Check sheet for the drawn part. Datum: minimum x, y, z corner. Units: mm. A direction names the side the tool comes from. Round coordinates to 2 decimals unless told otherwise and drop trailing zeros. Write each loop counter-clockwise with the first axis right and the second up, starting at its lowest first coordinate (ties: lowest second). Pieces come first, ordered by that corner, then holes.
Item 1: Tool access check on the marked faces 1, 2 and 3. Record the directions out of +Z, -Z, +X, -X, +Y, -Y that give a thin tool (end or side, any length) a straight path to the whole face; none if there is none.
Item 2: Cross-section at C-C on x = 38. Enter the section's corners in (y, z).
Item 3: Cross-section at D-D on x = 26. Enter the section's corners in (y, z), plus the area to 3 significant figures.
Item 4: Material ranges on line 1 (Z direction, x = 45, y = 4.75); line 2 (X direction, y = 4.5, z = 25.75), recorded low to high.
Item 5: Go/stop test with flat-tipped pins: pin 1 Ø10 at (y, z) = (10.5, 17.5) entering from +X; pin 2 Ø2 at (y, z) = (10.5, 13.5) entering from -X; pin 3 Ø0.5 at (y, z) = (15, 27.5) entering from -X. Record where each tip stops, or that it passes through.
Item 6: Cross-section at A-A on y = 18.5. Enter the section's corners in (x, z).
Item 7: Cross-section at B-B on z = 14.5. Enter the section's corners in (x, y).
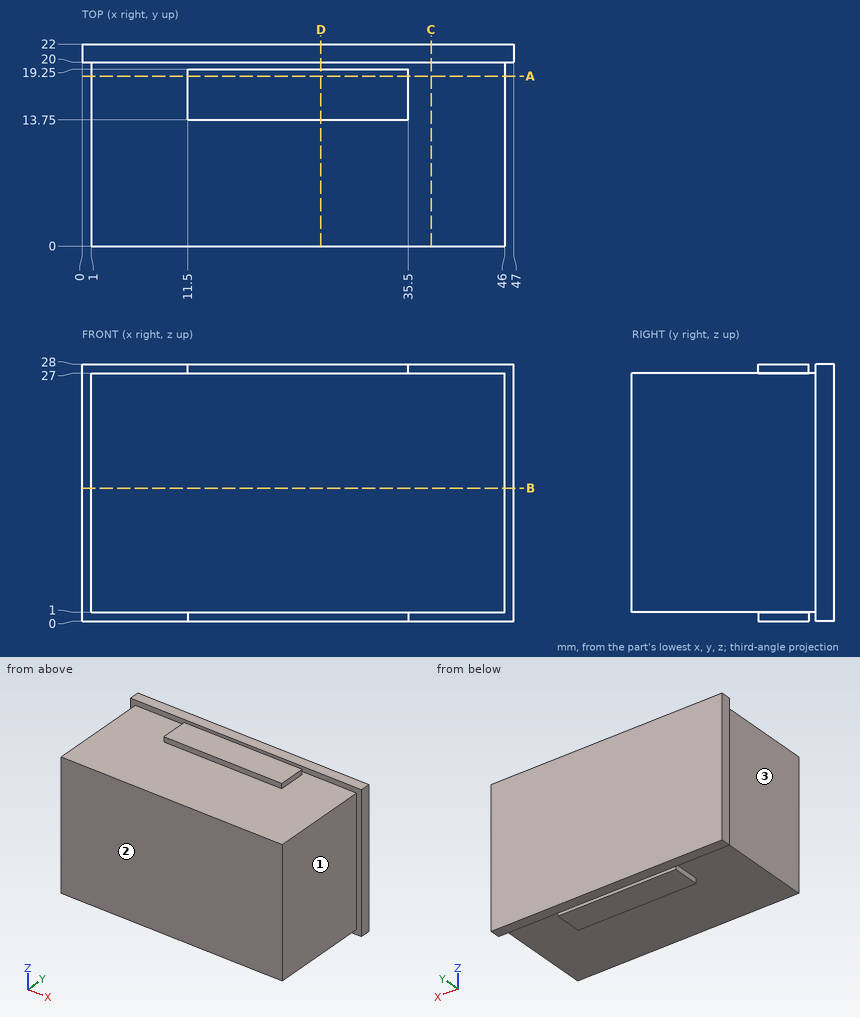
Response values:
1. face 1: +Z, -Z, +X, -Y
1. face 2: +Z, -Z, +X, -X, -Y
1. face 3: +Z, -Z, -X, -Y
2. outline: (0, 1) - (20, 1) - (20, 0) - (22, 0) - (22, 28) - (20, 28) - (20, 27) - (0, 27) - close
3. outline: (0, 1) - (13.75, 1) - (13.75, 0) - (19.25, 0) - (19.25, 1) - (20, 1) - (20, 0) - (22, 0) - (22, 28) - (20, 28) - (20, 27) - (19.25, 27) - (19.25, 28) - (13.75, 28) - (13.75, 27) - (0, 27) - close
3. area: 587 mm2
4. line 1: z = 1 to 27
4. line 2: x = 1 to 46
5. pin 1: stops at x = 46
5. pin 2: stops at x = 1
5. pin 3: stops at x = 11.5
6. outline: (1, 1) - (11.5, 1) - (11.5, 0) - (35.5, 0) - (35.5, 1) - (46, 1) - (46, 27) - (35.5, 27) - (35.5, 28) - (11.5, 28) - (11.5, 27) - (1, 27) - close
7. outline: (0, 20) - (1, 20) - (1, 0) - (46, 0) - (46, 20) - (47, 20) - (47, 22) - (0, 22) - close
